Source: CAD feature listing. Evaluate the final solid. Frame: model axes, mm. A direction names the side the tool comes from. Coordinates: 2 decimals unless noted, no trailing zeros. Loops run counter-clockwise (first coordinate to the right, second up) from the corner with the lowest first, then second, coordinate; pieces in that order, holes last.
from build123d import *

# Parameters (mm, degrees)
SKETCH1_W                                = 231.5
SKETCH1_H                                = 201.5
SKETCH1_W_2                              = 210.5
SKETCH1_H_2                              = 180.5
MAIN_BODY_DEPTH                          = 6
FILLET1_R                                = 5
FILLET2_R                                = 6
SKETCH3_W                                = 227.5
SKETCH3_H                                = 197.5
SKETCH3_W_2                              = 214
SKETCH3_H_2                              = 184
MAIN_CAVITY_DEPTH                        = 5
FILLET6_R                                = 6
FILLET4_R                                = 5
CAVITY1_START                            = 83.43860018
CAVITY1_OUTLINE_W                        = 1.804040507
CAVITY1_OUTLINE_H                        = 10
CAVITY1_DEPTH                            = 1.060660172
CAVITY1_START_2                          = -80.256619665
CAVITY1_2_OUTLINE_W                      = 1.56139982
CAVITY1_2_OUTLINE_H                      = 10
CAVITY1_2_DEPTH                          = 1.060660172
SNAP_START                               = -0.4
SNAP_FIT_DEPTH                           = 10.8
MIRROR1_START                            = -0.4
MIRROR1_AT_THE_SECOND_PLANE_COPY_1_DEPTH = 10.8
FILLET7_R                                = 0.5


# Read off the part's stored shape, not the designer's step: Cavity1
with BuildPart() as part:
    # Sketch1 → Main Body (new body)
    with BuildSketch(Plane.XY):
        Rectangle(SKETCH1_W, SKETCH1_H)
        Rectangle(SKETCH1_W_2, SKETCH1_H_2, mode=Mode.SUBTRACT)
    extrude(amount=MAIN_BODY_DEPTH)

    # Fillet1
    fillet1_edges = [part.edges().sort_by_distance(p)[0] for p in [
        (105.25, -90.25, 3),
        (105.25, 90.25, 3),
        (-105.25, 90.25, 3),
        (-105.25, -90.25, 3),
    ]]
    fillet(fillet1_edges, radius=FILLET1_R)

    # Fillet2
    fillet2_edges = [part.edges().sort_by_distance(p)[0] for p in [
        (115.75, -100.75, 3),
        (-115.75, -100.75, 3),
        (-115.75, 100.75, 3),
        (115.75, 100.75, 3),
    ]]
    fillet(fillet2_edges, radius=FILLET2_R)

    # Sketch3 → Main Cavity (cut)
    with BuildSketch(Plane(origin=(0, 0, 0), x_dir=(-1, 0, 0), z_dir=(0, 0, -1))):
        Rectangle(SKETCH3_W, SKETCH3_H)
        Rectangle(SKETCH3_W_2, SKETCH3_H_2, mode=Mode.SUBTRACT)
    extrude(amount=-MAIN_CAVITY_DEPTH, mode=Mode.SUBTRACT)

    # Fillet6
    fillet6_edges = [part.edges().sort_by_distance(p)[0] for p in [
        (-113.75, 98.75, 2.5),
        (-113.75, -98.75, 2.5),
        (113.75, -98.75, 2.5),
        (113.75, 98.75, 2.5),
    ]]
    fillet(fillet6_edges, radius=FILLET6_R)

    # Fillet4
    fillet4_edges = [part.edges().sort_by_distance(p)[0] for p in [
        (-107, -92, 2.5),
        (107, -92, 2.5),
        (107, 92, 2.5),
        (-107, 92, 2.5),
    ]]
    fillet(fillet4_edges, radius=FILLET4_R)

    # Cavity1 outline → Cavity1 (cut)
    with BuildSketch(Plane(origin=(0, 0, 0), x_dir=(0.7071067811865474, 0, -0.7071067811865477), z_dir=(0.7071067811865476, 0, 0.7071067811865476)).offset(CAVITY1_START)):
        with Locations((80.097979747, 65)):
            Rectangle(CAVITY1_OUTLINE_W, CAVITY1_OUTLINE_H)
        with Locations((80.097979747, -65)):
            Rectangle(CAVITY1_OUTLINE_W, CAVITY1_OUTLINE_H)
    extrude(amount=CAVITY1_DEPTH, mode=Mode.SUBTRACT)

    # Cavity1 2 outline → Cavity1 2 (cut)
    with BuildSketch(Plane(origin=(0, 0, 0), x_dir=(0.7071067811865474, 0, -0.7071067811865477), z_dir=(0.7071067811865476, 0, 0.7071067811865476)).offset(CAVITY1_START_2)):
        with Locations((-84.21930009, 65)):
            Rectangle(CAVITY1_2_OUTLINE_W, CAVITY1_2_OUTLINE_H)
        with Locations((-84.21930009, -65)):
            Rectangle(CAVITY1_2_OUTLINE_W, CAVITY1_2_OUTLINE_H)
    extrude(amount=CAVITY1_2_DEPTH, mode=Mode.SUBTRACT)

    # Sketch4 → Snap Fit (cut)
    with BuildSketch(Plane.XZ.offset(-70).offset(SNAP_START)):
        Polygon((-115.75, 4.315685425), (-114.575735931, 3.141421356), (-115.75, 1.967157288), align=None)
    snap_fit = extrude(amount=SNAP_FIT_DEPTH, mode=Mode.SUBTRACT)

    # Mirror1: Snap Fit across plane
    add(snap_fit.mirror(Plane.ZX), mode=Mode.SUBTRACT)

    # Mirror1 at the second plane: Snap Fit across plane
    add(snap_fit.mirror(Plane(origin=(0, 0, 0), x_dir=(0, 0, 1), z_dir=(1, 0, 0))), mode=Mode.SUBTRACT)

    # Mirror1 at the second plane copy 1 sketc → Mirror1 at the second plane copy 1 (cut)
    with BuildSketch(Plane(origin=(0, -70, 0), x_dir=(-1, 0, 0), z_dir=(0, 1, 0)).offset(MIRROR1_START)):
        Polygon((-115.75, 4.315685425), (-114.575735931, 3.141421356), (-115.75, 1.967157288), align=None)
    extrude(amount=MIRROR1_AT_THE_SECOND_PLANE_COPY_1_DEPTH, mode=Mode.SUBTRACT)

    # Fillet7
    fillet7_edges = [part.edges().sort_by_distance(p)[0] for p in [
        (-113.75, 0, 5),
        (0, -98.75, 5),
        (0, 98.75, 5),
        (113.75, 0, 5),
        (-111.992640687, 96.992640687, 5),
        (111.992640687, 96.992640687, 5),
        (111.992640687, -96.992640687, 5),
        (-111.992640687, -96.992640687, 5),
        (107, 0, 5),
        (0, -92, 5),
        (0, 92, 5),
        (-107, 0, 5),
        (105.535533906, -90.535533906, 5),
        (105.535533906, 90.535533906, 5),
        (-105.535533906, 90.535533906, 5),
        (-105.535533906, -90.535533906, 5),
        (105.25, 0, 6),
        (0, 90.25, 6),
        (0, -90.25, 6),
        (-105.25, 0, 6),
        (103.785533906, 88.785533906, 6),
        (103.785533906, -88.785533906, 6),
        (-103.785533906, -88.785533906, 6),
        (-103.785533906, 88.785533906, 6),
        (0, 100.75, 6),
        (115.75, 0, 6),
        (-115.75, 0, 6),
        (0, -100.75, 6),
        (-113.992640687, 98.992640687, 6),
        (-113.992640687, -98.992640687, 6),
        (113.992640687, -98.992640687, 6),
        (113.992640687, 98.992640687, 6),
    ]]
    fillet(fillet7_edges, radius=FILLET7_R)


solid = part.part
Q1. Section A-A, the plane y = -1.5. Return the cut outline in (x, z).
Q2. Contact query for flat-ended pins moving along their axis: pin 1 Ø1.3 at (x, z) = (-115, 3) entering from -Y; pin 2 Ø0.9 at (x, z) = (115.5, 2.5) entering from -Y; pin 3 Ø0.9 at (x, z) = (-115, 3.5) entering from -Y. Output: stop coordinate, or through.
Q3. Section B-B, the plane x = 34.5. Return the cut outline in (y, z).
Q4. Access query for faces 5 (the cylindrical face through (-112.039, -96.946, 2.282)), 6 (the cylindrical face through (113.946, -99.039, 2.788)), 7 (the cylindrical face through (-103.75, -88.82, 2.79)). Directions: +Z, -Z, +X, -X, +Y, -Y. A direction counts if a zero-diameter tool reaches every point of the face in a straight line with its end or side. Return the directions, or none.
Q5. Draft query along Y for faces 1 (the flat face through (-2, 100.75, 3)), 2 (the flat face through (105.25, -1, 3)), 3 (the cylindrical face through (105, 91, 2)), 4 (the flat face through (-2, -100.75, 3)). Return one class per face: +Y half, -Y half, draft (parallel to the pull), parting line (faces both ways), or undercut.
Q6. Line query: line 1 along X through (y, z) = (-14.5, 2); line 2 along Y through (x, z) = (-45.5, 2.7). Output: solid intervals per line, ascending.
Derived:
1. outline: (-115.75, 0) - (-113.75, 0) - (-113.75, 4.5) arc R0.5 cw to (-113.25, 5) - (-107.5, 5) arc R0.5 cw to (-107, 4.5) - (-107, 0) - (-105.25, 0) - (-105.25, 5.5) arc R0.5 ccw to (-105.75, 6) - (-115.25, 6) arc R0.5 ccw to (-115.75, 5.5) - close; (105.25, 0) - (107, 0) - (107, 4.5) arc R0.5 cw to (107.5, 5) - (113.25, 5) arc R0.5 cw to (113.75, 4.5) - (113.75, 0) - (115.75, 0) - (115.75, 5.5) arc R0.5 ccw to (115.25, 6) - (105.75, 6) arc R0.5 ccw to (105.25, 5.5) - close
2. pin 1: stops at y = -98.6
2. pin 2: stops at y = -97.56
2. pin 3: stops at y = -98.35
3. outline: (-100.75, 0) - (-98.75, 0) - (-98.75, 4.5) arc R0.5 cw to (-98.25, 5) - (-92.5, 5) arc R0.5 cw to (-92, 4.5) - (-92, 0) - (-90.25, 0) - (-90.25, 5.5) arc R0.5 ccw to (-90.75, 6) - (-100.25, 6) arc R0.5 ccw to (-100.75, 5.5) - close; (90.25, 0) - (92, 0) - (92, 4.5) arc R0.5 cw to (92.5, 5) - (98.25, 5) arc R0.5 cw to (98.75, 4.5) - (98.75, 0) - (100.75, 0) - (100.75, 5.5) arc R0.5 ccw to (100.25, 6) - (90.75, 6) arc R0.5 ccw to (90.25, 5.5) - close
4. face 5: -Z
4. face 6: +Z, -Z, +X, -Y
4. face 7: +Z, -Z
5. face 1: +Y half
5. face 2: undercut
5. face 3: undercut
5. face 4: -Y half
6. line 1: x = -115.75 to -113.75, -107 to -105.25, 105.25 to 107, 113.75 to 115.75
6. line 2: y = -100.75 to -98.75, -92 to -90.25, 90.25 to 92, 98.75 to 100.75
